Autodesk Inventor part; units mm, degrees
ref_plane "YZ Plane" through (0, 0, 0) normal (1, 0, 0) x (0, 1, 0)
ref_plane "XZ Plane" through (0, 0, 0) normal (0, 1, 0) x (-1, 0, 0)
ref_plane "XY Plane" through (0, 0, 0) normal (0, 0, 1) x (1, 0, 0)
sketch "Szkic1" plane through (0, 0, 0) normal (1, 0, 0) x (0, 1, 0)
  circle A0 centre (0, 0) radius 10
  line L0 (-14, 0) -> (14, 0)
  line L1 (0, -20) -> (0, 15)
  line L2 (10, 0) -> (10, -15)
  line L3 (-10, -15) -> (10, -15)
  line L4 (-10, 0) -> (-10, -15)
  dimension "d0" = 20
  dimension "d3" = 15
extrude "Wyciągnięcie proste2" add sketch "Szkic1" along normal blind 10
extrude "Wyciągnięcie proste3" add sketch "Szkic1" against normal blind 10 contours L0 L1 A0 | A0 L1 L0 | L1 L0 A0 | A0 L0 L1
sketch "Szkic2" plane through (-10, 0, 0) normal (-1, 0, 0) x (0, 0, 1)
  circle A0 centre (0, 0) radius 10
  circle A1 centre (0, 0) radius 8
  line L0 (-20, 0) -> (15, 0)
  line L1 (0, -14) -> (0, 14)
  circle A2 centre (-4, 0) radius 1
  circle A3 centre (4, 0) radius 1
  dimension "d8" = 16
  dimension "d9" = 2
  dimension "d12" = 8
extrude "Wyciągnięcie proste4" cut sketch "Szkic2" against normal blind 10 contours L0 A3 L1 A1 | A1 L1 L0 A3 | L1 L0 A2 A1 | A1 L0 A2 L1
extrude "Wyciągnięcie proste5" cut sketch "Szkic2" against normal blind 17 contours A3 L0 | L0 A3 | A2 L0 | L0 A2
equation "\"d12\" = 0.5 * d8"
properties part number "uchwytG5"
Could you check a few things on this model? Use its own coordinates, in mm. A direction names the side the tool comes from. Coordinates: 2 decimals unless noted, no trailing zeros. Write each loop counter-clockwise with the first axis right and the second up, starting at its lowest first coordinate (ties: lowest second). Pieces come first, ordered by that corner, then holes. Notation, with made-up numbers: (15, 5) - (33, 5) arc R17 ccw to (33, 12) - close; hole circle Ø4 at (30, 71.25). An arc over 180 degrees is marked (long way). Put each result on its own line as item: value. Start each with the question number.
Q1. I want a section at B-B on x = 4.25. Write out the boundary of the cut face in (y, z), plus the area to 3 significant figures.
Q2. I want a section at D-D on x = -8. Write out the boundary of the cut face in (y, z).
Q3. Thinking about a two-plate mould opening in Z: for faces 1 (the flat face through (5, 0, -15)), 2 (the flat face through (5, -10, -7)), 3 (the cylindrical face through (-5.07, -7.81, -1.73)), which applies, pulls with the +Z half, pulls with the -Z half, needs draft (parallel to the pull), parting line crosses it, or undercut?
Q4. Please list where these lines run through material, in increasing order: L1, parallel to Y at x = -2.75, z = 0; L2, parallel to Y at x = 3.5, z = -4.
Q5. I'm going to push flat-ended pins straight in: P1, Ø1, axis at y = 0, z = 4, coming from the -X side; P2, Ø1, axis at x = -5, z = -1.5, coming from the +Y side; P3, Ø9.5, axis at y = 0, z = 0, coming from the -X side. Where does each tip first touch, or does it pass through?
Q6. I want a section at C-C on z = -4. Write out the boundary of the cut face in (x, y), plus the area to 3 significant figures.
Q7. I want a section at A-A on y = 0. Write out the boundary of the cut face in (x, z), plus the area to 3 significant figures.
Q8. Which directions (+Z, -Z, +X, -X, +Y, -Y) give clear straight access to the entire face, cutting with the end or side of a thin tool? Please do faces 4 (the flat face through (7, 0, -4)), 5 (the flat face through (0, 0, -11)), 6 (the flat face through (10, 0, -2)).
Checks:
1. outline: (-10, -15) - (10, -15) - (10, 0) arc R10 ccw to (-10, 0) - close; hole circle Ø2 at (0, -4); hole circle Ø2 at (0, 4)
1. area: 451 mm²
2. outline: circle Ø20 at (0, 0); hole circle Ø16 at (0, 0)
3. face 1: pulls with the -Z half
3. face 2: needs draft
3. face 3: undercut
4. L1: -10 to -8, 8 to 10
4. L2: -10 to -1, 1 to 10
5. P1: x = 7
5. P2: y = 9.95
5. P3: x = 0
6. outline: (-10, -9.17) - (0, -9.17) - (0, -10) - (10, -10) - (10, 10) - (0, 10) - (0, 9.17) - (-10, 9.17) - (-10, 6.93) - (0, 6.93) - (0, 1) - (7, 1) - (7, -1) - (0, -1) - (0, -6.93) - (-10, -6.93) - close
6. area: 231 mm²
7. outline: (-10, -10) - (0, -10) - (0, -15) - (10, -15) - (10, 10) - (-10, 10) - (-10, 8) - (0, 8) - (0, 5) - (7, 5) - (7, 3) - (0, 3) - (0, -3) - (7, -3) - (7, -5) - (0, -5) - (0, -8) - (-10, -8) - close
7. area: 262 mm²
8. face 4: -X
8. face 5: -Z, -X
8. face 6: +Z, -Z, +X, +Y, -Y
